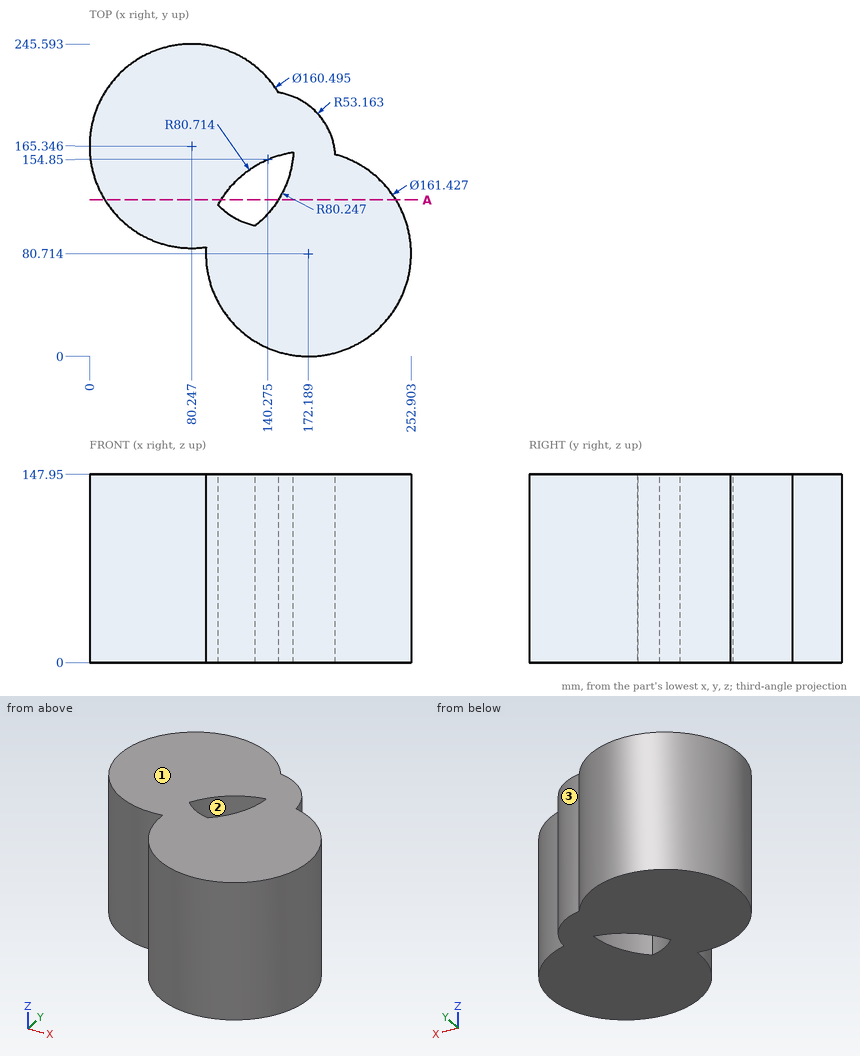
Design review of the part shown in the three views and the two pictorial views. Dimensions are in mm from the part's minimum x, y and z. Round coordinates to 2 decimals unless told otherwise and drop trailing zeros. Write each loop counter-clockwise with the first axis right and the second up, starting at its lowest first coordinate (ties: lowest second). Pieces come first, ordered by that corner, then holes. Notation, with made-up numbers: (66.25, -27) -> (96.25, -27) arc R25 ccw to (96.25, -7) -> close; hole circle Ø4 at (-36, 86.25). An arc over 180 degrees is marked (long way). Write item = value, one per line. Start each with the question number.
1) Take a section at A-A, the plane y = 123. State the section outline as (x, z) points.
2) Mouldability with a two-part tool opening along X and no side actions: class the marked faces 1, 2 and 3 as +X half, -X half, draft (parallel to the pull), parting line (faces both ways), or undercut.
3) Wall thickness on probe 1 along Y at (x, z) = (141, 50.5) (1 decimal); probe 2 along X at (y, z) = (83, 93); probe 3 along Y at (x, z) = (66, 77.5): over which ranges is each line inside the solid? List them lowest first. Write a range as from..to.
4) Clearance check with flat-ended pins moving along their axes: pin 1 (8 mm diameter, centred on x = 214.5, z = 67.5, fed in from -Y); pin 2 (8 mm diameter, centred on y = 25, z = 104.5, fed in from -X); pin 3 (6 mm diameter, centred on y = 55, z = 124.5, fed in from -X). State where each tip first meets the part, or that it passes through.
Results list:
q1.outline = (12.08, 0) -> (103.44, 0) -> (103.44, 147.95) -> (12.08, 147.95) -> close; (148.41, 0) -> (240.94, 0) -> (240.94, 147.95) -> (148.41, 147.95) -> close
q2.face_1 = draft
q2.face_2 = undercut
q2.face_3 = +X half
q3.probe_1 = 6.3..112.9, 155.2..217.8
q3.probe_2 = 91.51..252.87
q3.probe_3 = 86.37..244.32
q4.pin_1 = 9.67
q4.pin_2 = 110.22
q4.pin_3 = 94.74
